Part model, mm, in its own coordinate system. Give positions to 0.01 mm unless a question says otherwise; leave off trailing zeros. Order: outer loops, then holes, each group sorted by start corner. A loop starts at its lowest first (then second) coordinate and runs counter-clockwise, first axis right, second up. Notation, with made-up numbers: (-36.75, -39.75) -> (11.25, -39.75) arc R22 ccw to (11.25, -3.75) -> close; hole circle Ø3 at (56.5, -28.5). An arc over 180 degrees is marked (long way). Write item = value, one per line. Start each with the question number.
Item 1: Drill centre lines: line 1 along Z through (x, y) = (1.75, 32.5); line 2 along Z through (x, y) = (2, 52). Where is each one in solid material? Low to high.
Item 2: Flat gauge pin, fed straight in: P1, Ø1, axis at x = 2.5, z = 0, coming from the -Y side. Where does the tip first touch, or does it go through?
Item 3: Band-saw the part on A-A on y = 12. Write the cut outline in (x, z) (1 decimal), plus the area to 3 significant figures.
Autodesk Inventor part; units mm, degrees
ref_plane "YZ Plane" through (0, 0, 0) normal (1, 0, 0) x (0, 1, 0)
ref_plane "XZ Plane" through (0, 0, 0) normal (0, 1, 0) x (-1, 0, 0)
ref_plane "XY Plane" through (0, 0, 0) normal (0, 0, 1) x (1, 0, 0)
sketch "Sketch1" plane through (0, 0, 0) normal (0, 1, 0) x (-1, 0, 0)
  line L0 (3.175, -3.175) -> (-3.175, -3.175)
  line L1 (-3.175, -3.175) -> (-3.175, 3.175)
  line L2 (-3.175, 3.175) -> (3.175, 3.175)
  line L3 (3.175, 3.175) -> (3.175, -3.175)
  line L4 (3.175, -3.175) -> (-3.175, 3.175) construction
  line L5 (-3.175, -3.175) -> (3.175, 3.175) construction
  point P0 (0, 0)
  dimension "d0" = 6.35
  dimension "d1" = 6.35
extrude "Extrusion1" add sketch "Sketch1" along normal blind 101.6
fillet "Fillet1" radius 1.5875 4 edges at (3.175, 50.8, -3.175) (3.175, 50.8, 3.175) (-3.175, 50.8, -3.175) (-3.175, 50.8, 3.175)
fillet "Fillet2" radius 0.7937 16 edges at (3.175, 0, 0) (2.71, 0, -2.71) (0, 0, -3.175) (-2.71, 0, -2.71) (-3.175, 0, 0) (-2.71, 0, 2.71) (0, 0, 3.175) (2.71, 0, 2.71) (2.71, 101.6, -2.71) (0, 101.6, -3.175) (-2.71, 101.6, -2.71) (-3.175, 101.6, 0) (-2.71, 101.6, 2.71) (0, 101.6, 3.175) (2.71, 101.6, 2.71) (3.175, 101.6, 0)
properties part number "4 inch" material "Stainless Steel"
Values found:
q1.line_1 = -3.17 to 3.17
q1.line_2 = -3.12 to 3.12
q2.P1 = 0
q3.outline = (-3.2, -1.6) arc R1.6 ccw to (-1.6, -3.2) -> (1.6, -3.2) arc R1.6 ccw to (3.2, -1.6) -> (3.2, 1.6) arc R1.6 ccw to (1.6, 3.2) -> (-1.6, 3.2) arc R1.6 ccw to (-3.2, 1.6) -> close
q3.area = 38.2 mm^2
